The listing builds one solid part. Answer for the finished solid, in the listing's coordinates (mm). Face numbers are marked on the shaded views. A direction names the side the tool comes from. Give positions to 0.01 mm unless a question says otherwise; leave off trailing zeros. Order: outer loops, then holes, each group sorted by start corner. A loop starts at its lowest first (then second) coordinate and runs counter-clockwise, first axis right, second up.
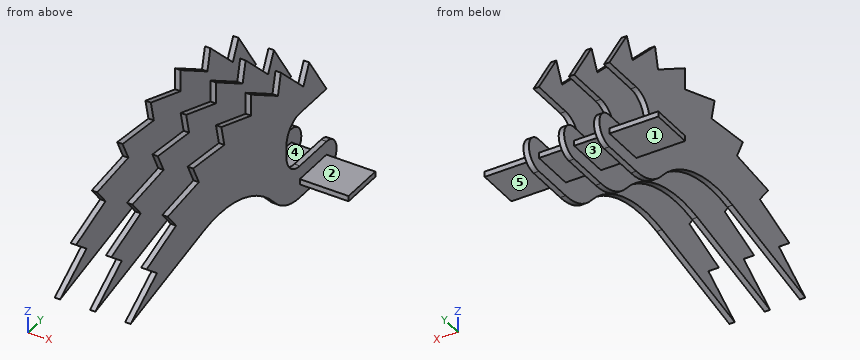
```python
from build123d import *

# Parameters (mm, degrees)
F1_DEPTH      = 1.5875
F1_DEPTH_BACK = 1.5875
F2_START      = 17.4625
F2_DEPTH      = 3.175
F3_START      = 17.4625
F3_DEPTH      = 3.175
F4_W          = 25.4
F4_H          = 3.175
F5_DEPTH      = 50.8
F5_DEPTH_BACK = 50.8


with BuildPart() as f1:
    # F0 (on Right) → F1 (new body, two sides)
    with BuildSketch(Plane.YZ) as f1_sk:
        with BuildLine():
            Line((-89.3638715037, 71.2642159143), (-114.423321003, 55.102664279))
            Line((-114.423321003, 55.102664279), (-45.394477118, 70.8098596439))
            ThreePointArc((-45.394477118, 70.8098596439), (-8.5270592577, 69.1620720095), (22.3122345378, 48.8923985547))
            ThreePointArc((22.3122345378, 48.8923985547), (33.0733487312, 40.9236595167), (46.1626316513, 38.0999999807))
            Line((46.1626316513, 38.0999999807), (71.5626337911, 38.0999999807))
            ThreePointArc((71.5626337911, 38.0999999807), (81.0876337911, 47.6249999807), (71.5626337911, 57.1499999807))
            Line((71.5626337911, 57.1499999807), (46.1626316513, 57.1499999807))
            ThreePointArc((46.1626316513, 57.1499999807), (37.1823755302, 60.8697438596), (33.4626316513, 69.8499999807))
            Line((33.4626316513, 69.8499999807), (33.4626316513, 76.1999999807))
            ThreePointArc((33.4626316513, 76.1999999807), (37.1823762868, 85.1802568583), (46.1626337911, 88.8999999807))
            Line((46.1626337911, 88.8999999807), (71.5626337911, 88.8999999807))
            Line((71.5626337911, 88.8999999807), (71.2626562096, 89.3651152853))
            Line((71.2626562096, 89.3651152853), (55.1006672069, 114.4242827085))
            Line((55.1006672069, 114.4242827085), (49.5906004862, 102.9818544376))
            Line((49.5906004862, 102.9818544376), (28.2576888992, 123.8164085171))
            Line((28.2576888992, 123.8164085171), (25.4319200093, 111.4347676654))
            Line((25.4319200093, 111.4347676654), (-0.0022165681, 126.9999999807))
            Line((-0.0022165681, 126.9999999807), (-0.0019949113, 114.2999999826))
            Line((-0.0019949113, 114.2999999826), (-28.26201089, 123.8154220623))
            Line((-28.26201089, 123.8154220623), (-25.435809801, 111.433879856))
            Line((-25.435809801, 111.433879856), (-55.1046613343, 114.4223592627))
            Line((-55.1046613343, 114.4223592627), (-49.5941952009, 102.9801233364))
            Line((-49.5941952009, 102.9801233364), (-79.184195108, 99.2918085499))
            Line((-79.184195108, 99.2918085499), (-71.2657755972, 89.3626276949))
            Line((-71.2657755972, 89.3626276949), (-99.2931905596, 79.1824621269))
            Line((-99.2931905596, 79.1824621269), (-89.3638715037, 71.2642159143))
        make_face()
    extrude(amount=F1_DEPTH)
    extrude(f1_sk.sketch, amount=-F1_DEPTH_BACK)



with BuildPart() as f2:
    # F1_face (on face) → F2 (new body)
    with BuildSketch(Plane(origin=(1.5875, -4.3675464113, 83.8957908955), x_dir=(0, 1, 0), z_dir=(1, 0, 0)).offset(F2_START)):
        with BuildLine():
            Line((-94.9256441483, -4.7133287685), (-84.9963250924, -12.6315749812))
            Line((-84.9963250924, -12.6315749812), (-110.0557745917, -28.7931266165))
            Line((-110.0557745917, -28.7931266165), (-41.0269307067, -13.0859312515))
            ThreePointArc((-41.0269307067, -13.0859312515), (-4.1595128464, -14.733718886), (26.6797809491, -35.0033923408))
            ThreePointArc((26.6797809491, -35.0033923408), (37.4408951425, -42.9721313788), (50.5301780626, -45.7957909148))
            Line((50.5301780626, -45.7957909148), (75.9301802024, -45.7957909148))
            ThreePointArc((75.9301802024, -45.7957909148), (85.4551802024, -36.2707909148), (75.9301802024, -26.7457909148))
            Line((75.9301802024, -26.7457909148), (50.5301780626, -26.7457909148))
            ThreePointArc((50.5301780626, -26.7457909148), (41.5499219415, -23.0260470359), (37.8301780626, -14.0457909148))
            Line((37.8301780626, -14.0457909148), (37.8301780626, -7.6957909148))
            ThreePointArc((37.8301780626, -7.6957909148), (41.5499226981, 1.2844659628), (50.5301802024, 5.0042090852))
            Line((50.5301802024, 5.0042090852), (75.9301802024, 5.0042090852))
            Line((75.9301802024, 5.0042090852), (59.4682136182, 30.528491813))
            Line((59.4682136182, 30.528491813), (53.9581468975, 19.0860635422))
            Line((53.9581468975, 19.0860635422), (32.6252353105, 39.9206176217))
            Line((32.6252353105, 39.9206176217), (29.7994664206, 27.5389767699))
            Line((29.7994664206, 27.5389767699), (4.3653298432, 43.1042090852))
            Line((4.3653298432, 43.1042090852), (4.3655515, 30.4042090871))
            Line((4.3655515, 30.4042090871), (-23.8944644787, 39.9196311668))
            Line((-23.8944644787, 39.9196311668), (-21.0682633897, 27.5380889606))
            Line((-21.0682633897, 27.5380889606), (-50.737114923, 30.5265683672))
            Line((-50.737114923, 30.5265683672), (-45.2266487895, 19.0843324409))
            Line((-45.2266487895, 19.0843324409), (-74.8166486967, 15.3960176544))
            Line((-74.8166486967, 15.3960176544), (-66.8982291859, 5.4668367994))
            Line((-66.8982291859, 5.4668367994), (-94.9256441483, -4.7133287685))
        make_face()
    extrude(amount=F2_DEPTH)


with BuildPart() as f3:
    # F1_face1 (on face) → F3 (new body)
    with BuildSketch(Plane(origin=(-1.5875, -4.3675464113, 83.8957908955), x_dir=(0, 1, 0), z_dir=(-1, 0, 0)).offset(F3_START)):
        with BuildLine():
            Line((-84.9963250924, 12.6315749812), (-94.9256441483, 4.7133287685))
            Line((-94.9256441483, 4.7133287685), (-66.8982291859, -5.4668367994))
            Line((-66.8982291859, -5.4668367994), (-74.8166486967, -15.3960176544))
            Line((-74.8166486967, -15.3960176544), (-45.2266487895, -19.0843324409))
            Line((-45.2266487895, -19.0843324409), (-50.737114923, -30.5265683672))
            Line((-50.737114923, -30.5265683672), (-21.0682633897, -27.5380889606))
            Line((-21.0682633897, -27.5380889606), (-23.8944644787, -39.9196311668))
            Line((-23.8944644787, -39.9196311668), (4.3655515, -30.4042090871))
            Line((4.3655515, -30.4042090871), (4.3653298432, -43.1042090852))
            Line((4.3653298432, -43.1042090852), (29.7994664206, -27.5389767699))
            Line((29.7994664206, -27.5389767699), (32.6252353105, -39.9206176217))
            Line((32.6252353105, -39.9206176217), (53.9581468975, -19.0860635422))
            Line((53.9581468975, -19.0860635422), (59.4682136182, -30.528491813))
            Line((59.4682136182, -30.528491813), (75.9301802024, -5.0042090852))
            Line((75.9301802024, -5.0042090852), (50.5301802024, -5.0042090852))
            ThreePointArc((50.5301802024, -5.0042090852), (41.5499226981, -1.2844659628), (37.8301780626, 7.6957909148))
            Line((37.8301780626, 7.6957909148), (37.8301780626, 14.0457909148))
            ThreePointArc((37.8301780626, 14.0457909148), (41.5499219415, 23.0260470359), (50.5301780626, 26.7457909148))
            Line((50.5301780626, 26.7457909148), (75.9301802024, 26.7457909148))
            ThreePointArc((75.9301802024, 26.7457909148), (85.4551802024, 36.2707909148), (75.9301802024, 45.7957909148))
            Line((75.9301802024, 45.7957909148), (50.5301780626, 45.7957909148))
            ThreePointArc((50.5301780626, 45.7957909148), (37.4408951425, 42.9721313788), (26.6797809491, 35.0033923408))
            ThreePointArc((26.6797809491, 35.0033923408), (-4.1595128464, 14.733718886), (-41.0269307067, 13.0859312515))
            Line((-41.0269307067, 13.0859312515), (-110.0557745917, 28.7931266165))
            Line((-110.0557745917, 28.7931266165), (-84.9963250924, 12.6315749812))
        make_face()
    extrude(amount=F3_DEPTH)


with BuildPart() as f1_1:
    add(f1.part)

    add(f2.part)  # F5 merges F2

    add(f3.part)  # F5 merges F3
    # F4 (on face) → F5 (join, two sides)
    with BuildSketch(Plane.YZ) as f5_sk:
        with Locations((58.8626337911, 47.6249999807)):
            Rectangle(F4_W, F4_H)
    extrude(amount=F5_DEPTH)
    extrude(f5_sk.sketch, amount=-F5_DEPTH_BACK)


solid = f1_1.part
```
1) A tool of negligible diameter and unlimited length cuts with its end or side. For the marked faces 1, 2 and 3, from which of +Z, -Z, +X, -X, +Y, -Y can it reach the whole face along a straight path? Write none if from no direction.
Geometry says:
face 1: -Z, -X, +Y, -Y
face 2: +Z, +X, +Y, -Y
face 3: -Z, +Y, -Y
2) Straight lines are drawn through the part: probe 1 along Z at (x, y) = (-33, 68); probe 2 along Z at (x, y) = (-21, -86.5). For each, find the intervals that lie inside material, in ascending order.
Geometry says:
probe 1: z = 46.04 to 49.21
probe 2: z = 61.46 to 83.83
3) For a pull along X with two mould halves and no side action, classify the marked faces 4 and 5 as +X half, -X half, draft (parallel to the pull), parting line (faces both ways), or undercut.
Geometry says:
face 4: undercut
face 5: draft
4) Find section A-A (z = 65). Count the separate pieces of the cut face and the enclosed holes in it, then the cut area to 3 significant figures.
Geometry says:
separate pieces: 6
enclosed holes: 0
area: 581 mm2
5) Given P1, Ø4, axis at x = 22, y = -62.5, coming from the +Z side; P2, Ø2.5, axis at x = -21, z = 72, coming from the +Y side; P3, Ø8.5, axis at x = -12, y = 62, coming from the -Z side, each flat-ended and moving along its own axis, determine where each tip first touches the part or whether it passes through.
Geometry says:
P1: stops at z = 101.62
P2: stops at y = 33.46
P3: stops at z = 46.04
6) Find section D-D (x = 8.5). Write down the section's boundary in (y, z).
Geometry says:
outline: (46.16, 46.04) - (71.56, 46.04) - (71.56, 49.21) - (46.16, 49.21) - close
